Here's how the part is built. I have some questions about the finished solid (model axes, mm). Face numbers are marked on the shaded views. Round coordinates to 2 decimals unless told otherwise and drop trailing zeros. Loops run counter-clockwise (first coordinate to the right, second up) from the corner with the lowest first, then second, coordinate; pieces in that order, holes last. Notation, with made-up numbers: (3, 0) -> (54, 0) arc R14 ccw to (54, 27) -> close; hole circle Ø7 at (7, 12.5). An arc over 180 degrees is marked (long way). One line per item, written item: value. Start each with the question number.
```python
from build123d import *

# Parameters (mm, degrees)
SKETCH1_R           = 21
BOSS_EXTRUDE1_DEPTH = 110
SKETCH2_R           = 160
BOSS_EXTRUDE2_DEPTH = 500
SKETCH3_W           = 320
SKETCH3_H           = 320
BOSS_EXTRUDE3_DEPTH = 15
SKETCH4_R           = 7.5
CUT_EXTRUDE1_DEPTH  = 15
CHAMFER1_SIZE       = 10
CUT_EXTRUDE2_DEPTH  = 5
SKETCH7_R           = 6
CUT_EXTRUDE3_DEPTH  = 50


with BuildPart() as part:
    # Sketch1 → Boss-Extrude1 (new body)
    with BuildSketch(Plane(origin=(0, 0, 0), x_dir=(0, 0, -1), z_dir=(1, 0, 0))):
        Circle(SKETCH1_R)
    extrude(amount=BOSS_EXTRUDE1_DEPTH)

    # Sketch2 → Boss-Extrude2 (add)
    with BuildSketch(Plane(origin=(110, 0, 0), x_dir=(0, 0, -1), z_dir=(1, 0, 0))):
        Circle(SKETCH2_R)
    extrude(amount=BOSS_EXTRUDE2_DEPTH)

    # Sketch3 → Boss-Extrude3 (add)
    with BuildSketch(Plane(origin=(0, -160, 0), x_dir=(1, 0, 0), z_dir=(0, 1, 0))):
        with Locations((300, 0)):
            Rectangle(SKETCH3_W, SKETCH3_H)
    extrude(amount=BOSS_EXTRUDE3_DEPTH)

    # Sketch4 → Cut-Extrude1 (cut)
    with BuildSketch(Plane.XZ.offset(160)):
        with Locations(Location((428, 127, 0), (0, 0, 270))):
            Circle(SKETCH4_R)
        with Locations(Location((218, 127, 0), (0, 0, 270))):
            Circle(SKETCH4_R)
        with Locations(Location((218, -127, 0), (0, 0, 270))):
            Circle(SKETCH4_R)
        with Locations(Location((428, -127, 0), (0, 0, 270))):
            Circle(SKETCH4_R)
    extrude(amount=-CUT_EXTRUDE1_DEPTH, mode=Mode.SUBTRACT)

    # Chamfer1
    chamfer1_edges = [part.edges().sort_by_distance(p)[0] for p in [
        (110, 0, 160),
        (610, 0, 160),
    ]]
    chamfer(chamfer1_edges, length=CHAMFER1_SIZE)

    # Sketch5 → Cut-Revolve1 (revolve, cut)
    with BuildSketch(Plane.XY, mode=Mode.PRIVATE) as cut_revolve1_sk:
        Polygon((145.021608212, 165.529428324), (110, 165.529428324), (110, 37.056137485), (115.568052014, 53.947048233), (126.316813399, 69.30242164), (136.897249661, 84.417330587), (136.897249661, 105.131626256), (145.021608212, 129.777196164), align=None)
    revolve(cut_revolve1_sk.sketch.rotate(Axis((0, 0, 0), (-1, 0, 0)), 90), axis=Axis((0, 0, 0), (-1, 0, 0)), mode=Mode.SUBTRACT)

    # Sketch6 → Cut-Extrude2 (cut)
    with BuildSketch(Plane(origin=(0, 21, 0), x_dir=(1, 0, 0), z_dir=(0, 1, 0))):
        with BuildLine():
            Line((104, 6), (0, 6))
            Line((0, 6), (0, -6))
            Line((0, -6), (104, -6))
            ThreePointArc((104, -6), (110, 0), (104, 6))
        make_face()
    extrude(amount=-CUT_EXTRUDE2_DEPTH, mode=Mode.SUBTRACT)

    # Sketch7 → Cut-Extrude3 (cut)
    with BuildSketch(Plane.ZY):
        Circle(SKETCH7_R)
    extrude(amount=-CUT_EXTRUDE3_DEPTH, mode=Mode.SUBTRACT)


solid = part.part
```
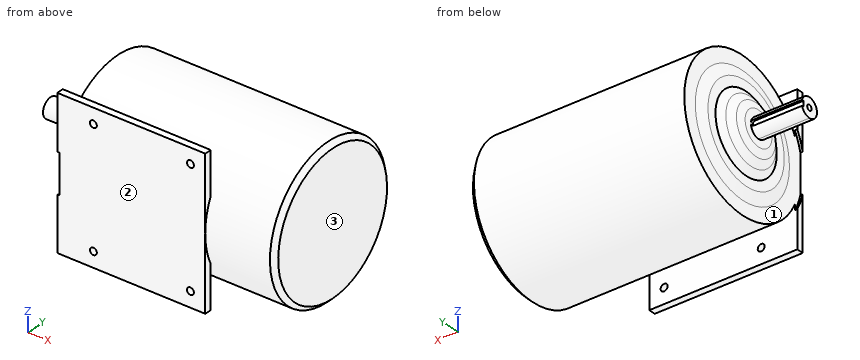
Q1. If I drill on line 1 along X through (y, z) = (-150.25, 127); line 2 along Y through (x, z) = (152, 106.5); line 3 along Z through (x, y) = (359, 1.5), over which ranges is the centre line in solid material (lowest first)?
Q2. If we mould it in two halves opening along Y, with no side actions, what happens to the marked faces 1, 2 and 3? For each: released by +Y, released by -Y, zero draft, split by the parting line, or undercut.
Q3. I want a section at A-A on x = 218. Please give me the cut outline in (y, z).
Q4. Will these pins go through, and if not, where does the flat tip stop? P1, Ø1.2, axis at x = 28.5, y = 17.5, coming from the +Z side; P2, Ø12, axis at y = -154.5, z = -80.5, coming from the -X side; P3, Ø7.5, axis at y = -151, z = -68, coming from the +X side.
Answers below:
1. line 1: x = 140 to 210.5, 225.5 to 420.5, 435.5 to 460
1. line 2: y = -160 to -145, -119.41 to 119.41
1. line 3: z = -159.99 to 159.99
2. face 1: undercut
2. face 2: released by -Y
2. face 3: zero draft
3. outline: (-160, -160) -> (-145, -160) -> (-145, -134.5) -> (-160, -134.5) -> close; (-160, -119.5) -> (-145, -119.5) -> (-145, -67.64) arc R160 ccw (long way) to (-145, 67.64) -> (-145, 119.5) -> (-160, 119.5) -> close; (-160, 134.5) -> (-145, 134.5) -> (-145, 160) -> (-160, 160) -> close
4. P1: stops at z = 12.47
4. P2: stops at x = 140
4. P3: stops at x = 460
